from build123d import *

# Parameters (mm, degrees)
SKETCH1_R           = 44.45
BOSS_EXTRUDE1_DEPTH = 10
BOSS_EXTRUDE2_DEPTH = 3
SKETCH3_R           = 5
CUT_EXTRUDE1_DEPTH  = 10
SKETCH4_R           = 5
SKETCH4_R_2         = 3.25
BOSS_EXTRUDE4_DEPTH = 3
CHAMFER1_SIZE       = 0.5


with BuildPart() as part:
    # Sketch1 → Boss-Extrude1 (new body)
    with BuildSketch(Plane(origin=(0, 0, 0), x_dir=(1, 0, 0), z_dir=(0, 1, 0))):
        with Locations(Location((0, 0, 0), (0, 0, 270))):
            Circle(SKETCH1_R)
        with BuildLine():
            ThreePointArc((37.087043144, 17.293972236), (28.935533906, 28.935533906), (17.293972236, 37.087043144))
            ThreePointArc((17.293972236, 37.087043144), (10.649341992, 34.668595517), (13.067789619, 28.023965273))
            ThreePointArc((13.067789619, 28.023965273), (21.864466094, 21.864466094), (28.023965273, 13.067789619))
            ThreePointArc((28.023965273, 13.067789619), (34.668595517, 10.649341992), (37.087043144, 17.293972236))
        make_face(mode=Mode.SUBTRACT)
        with BuildLine():
            ThreePointArc((17.293972236, -37.087043144), (28.935533906, -28.935533906), (37.087043144, -17.293972236))
            ThreePointArc((37.087043144, -17.293972236), (34.668595517, -10.649341992), (28.023965273, -13.067789619))
            ThreePointArc((28.023965273, -13.067789619), (21.864466094, -21.864466094), (13.067789619, -28.023965273))
            ThreePointArc((13.067789619, -28.023965273), (10.649341992, -34.668595517), (17.293972236, -37.087043144))
        make_face(mode=Mode.SUBTRACT)
        with BuildLine():
            ThreePointArc((-37.087043144, -17.293972236), (-28.935533906, -28.935533906), (-17.293972236, -37.087043144))
            ThreePointArc((-17.293972236, -37.087043144), (-10.649341992, -34.668595517), (-13.067789619, -28.023965273))
            ThreePointArc((-13.067789619, -28.023965273), (-21.864466094, -21.864466094), (-28.023965273, -13.067789619))
            ThreePointArc((-28.023965273, -13.067789619), (-34.668595517, -10.649341992), (-37.087043144, -17.293972236))
        make_face(mode=Mode.SUBTRACT)
        with BuildLine():
            ThreePointArc((-17.293972236, 37.087043144), (-28.935533906, 28.935533906), (-37.087043144, 17.293972236))
            ThreePointArc((-37.087043144, 17.293972236), (-34.668595517, 10.649341992), (-28.023965273, 13.067789619))
            ThreePointArc((-28.023965273, 13.067789619), (-21.864466094, 21.864466094), (-13.067789619, 28.023965273))
            ThreePointArc((-13.067789619, 28.023965273), (-10.649341992, 34.668595517), (-17.293972236, 37.087043144))
        make_face(mode=Mode.SUBTRACT)
    extrude(amount=BOSS_EXTRUDE1_DEPTH)

    # Sketch2 → Boss-Extrude2 (add)
    with BuildSketch(Plane(origin=(0, 10, 0), x_dir=(1, 0, 0), z_dir=(0, 1, 0))):
        with BuildLine():
            ThreePointArc((-17.293972236, 37.087043144), (-28.935533906, 28.935533906), (-37.087043144, 17.293972236))
            ThreePointArc((-37.087043144, 17.293972236), (-34.668595517, 10.649341992), (-28.023965273, 13.067789619))
            ThreePointArc((-28.023965273, 13.067789619), (-21.864466094, 21.864466094), (-13.067789619, 28.023965273))
            ThreePointArc((-13.067789619, 28.023965273), (-10.649341992, 34.668595517), (-17.293972236, 37.087043144))
        make_face()
        with BuildLine():
            ThreePointArc((-16.554390278, 35.501004516), (-12.23538062, 33.929013559), (-13.807371577, 29.610003901))
            ThreePointArc((-13.807371577, 29.610003901), (-23.101902961, 23.101902961), (-29.610003901, 13.807371577))
            ThreePointArc((-29.610003901, 13.807371577), (-33.929013559, 12.23538062), (-35.501004516, 16.554390278))
            ThreePointArc((-35.501004516, 16.554390278), (-27.698097039, 27.698097039), (-16.554390278, 35.501004516))
        make_face(mode=Mode.SUBTRACT)
        with BuildLine():
            ThreePointArc((17.293972236, 37.087043144), (10.649341992, 34.668595517), (13.067789619, 28.023965273))
            ThreePointArc((13.067789619, 28.023965273), (21.864466094, 21.864466094), (28.023965273, 13.067789619))
            ThreePointArc((28.023965273, 13.067789619), (34.668595517, 10.649341992), (37.087043144, 17.293972236))
            ThreePointArc((37.087043144, 17.293972236), (28.935533906, 28.935533906), (17.293972236, 37.087043144))
        make_face()
        with BuildLine():
            ThreePointArc((35.501004516, 16.554390278), (33.929013559, 12.23538062), (29.610003901, 13.807371577))
            ThreePointArc((29.610003901, 13.807371577), (23.101902961, 23.101902961), (13.807371577, 29.610003901))
            ThreePointArc((13.807371577, 29.610003901), (12.23538062, 33.929013559), (16.554390278, 35.501004516))
            ThreePointArc((16.554390278, 35.501004516), (27.698097039, 27.698097039), (35.501004516, 16.554390278))
        make_face(mode=Mode.SUBTRACT)
        with BuildLine():
            ThreePointArc((37.087043144, -17.293972236), (34.668595517, -10.649341992), (28.023965273, -13.067789619))
            ThreePointArc((28.023965273, -13.067789619), (21.864466094, -21.864466094), (13.067789619, -28.023965273))
            ThreePointArc((13.067789619, -28.023965273), (10.649341992, -34.668595517), (17.293972236, -37.087043144))
            ThreePointArc((17.293972236, -37.087043144), (28.935533906, -28.935533906), (37.087043144, -17.293972236))
        make_face()
        with BuildLine():
            ThreePointArc((16.554390278, -35.501004516), (12.23538062, -33.929013559), (13.807371577, -29.610003901))
            ThreePointArc((13.807371577, -29.610003901), (23.101902961, -23.101902961), (29.610003901, -13.807371577))
            ThreePointArc((29.610003901, -13.807371577), (33.929013559, -12.23538062), (35.501004516, -16.554390278))
            ThreePointArc((35.501004516, -16.554390278), (27.698097039, -27.698097039), (16.554390278, -35.501004516))
        make_face(mode=Mode.SUBTRACT)
        with BuildLine():
            ThreePointArc((-28.023965273, -13.067789619), (-34.668595517, -10.649341992), (-37.087043144, -17.293972236))
            ThreePointArc((-37.087043144, -17.293972236), (-28.935533906, -28.935533906), (-17.293972236, -37.087043144))
            ThreePointArc((-17.293972236, -37.087043144), (-10.649341992, -34.668595517), (-13.067789619, -28.023965273))
            ThreePointArc((-13.067789619, -28.023965273), (-21.864466094, -21.864466094), (-28.023965273, -13.067789619))
        make_face()
        with BuildLine():
            ThreePointArc((-35.501004516, -16.554390278), (-33.929013559, -12.23538062), (-29.610003901, -13.807371577))
            ThreePointArc((-29.610003901, -13.807371577), (-23.101902961, -23.101902961), (-13.807371577, -29.610003901))
            ThreePointArc((-13.807371577, -29.610003901), (-12.23538062, -33.929013559), (-16.554390278, -35.501004516))
            ThreePointArc((-16.554390278, -35.501004516), (-27.698097039, -27.698097039), (-35.501004516, -16.554390278))
        make_face(mode=Mode.SUBTRACT)
    extrude(amount=-BOSS_EXTRUDE2_DEPTH)

    # Sketch3 → Cut-Extrude1 (cut)
    with BuildSketch(Plane(origin=(0, 10, 0), x_dir=(1, 0, 0), z_dir=(0, 1, 0))):
        with Locations(Location((0, 14.664696837, 0), (0, 0, 270))):
            Circle(SKETCH3_R)
        with Locations(Location((-12.7, -7.332348419, 0), (0, 0, 270))):
            Circle(SKETCH3_R)
        with Locations(Location((12.7, -7.332348419, 0), (0, 0, 270))):
            Circle(SKETCH3_R)
    extrude(amount=-CUT_EXTRUDE1_DEPTH, mode=Mode.SUBTRACT)

    # Sketch4 → Boss-Extrude4 (add)
    with BuildSketch(Plane(origin=(0, 0, 0), x_dir=(1, 0, 0), z_dir=(0, 1, 0))):
        with Locations(Location((12.7, -7.332348419, 0), (0, 0, 270))):
            Circle(SKETCH4_R)
        with Locations(Location((12.7, -7.332348419, 0), (0, 0, 270))):
            Circle(SKETCH4_R_2, mode=Mode.SUBTRACT)
        with Locations(Location((-12.7, -7.332348419, 0), (0, 0, 270))):
            Circle(SKETCH4_R)
        with Locations(Location((-12.7, -7.332348419, 0), (0, 0, 270))):
            Circle(SKETCH4_R_2, mode=Mode.SUBTRACT)
        with Locations(Location((0, 14.664696837, 0), (0, 0, 270))):
            Circle(SKETCH4_R)
        with Locations(Location((0, 14.664696837, 0), (0, 0, 270))):
            Circle(SKETCH4_R_2, mode=Mode.SUBTRACT)
    extrude(amount=BOSS_EXTRUDE4_DEPTH)

    # Chamfer1
    chamfer1_edges = [part.edges().sort_by_distance(p)[0] for p in [
        (-34.668595517, 0, 10.649341992),
        (-28.935533906, 0, 28.935533906),
        (-10.649341992, 0, 34.668595517),
        (-21.864466094, 0, 21.864466094),
        (0, 0, -44.45),
        (10.649341992, 0, 34.668595517),
        (28.935533906, 0, 28.935533906),
        (34.668595517, 0, 10.649341992),
        (21.864466094, 0, 21.864466094),
        (-28.935533906, 0, -28.935533906),
        (-34.668595517, 0, -10.649341992),
        (-21.864466094, 0, -21.864466094),
        (-10.649341992, 0, -34.668595517),
        (34.668595517, 0, -10.649341992),
        (28.935533906, 0, -28.935533906),
        (10.649341992, 0, -34.668595517),
        (21.864466094, 0, -21.864466094),
        (0, 10, -44.45),
    ]]
    chamfer(chamfer1_edges, length=CHAMFER1_SIZE)


solid = part.part
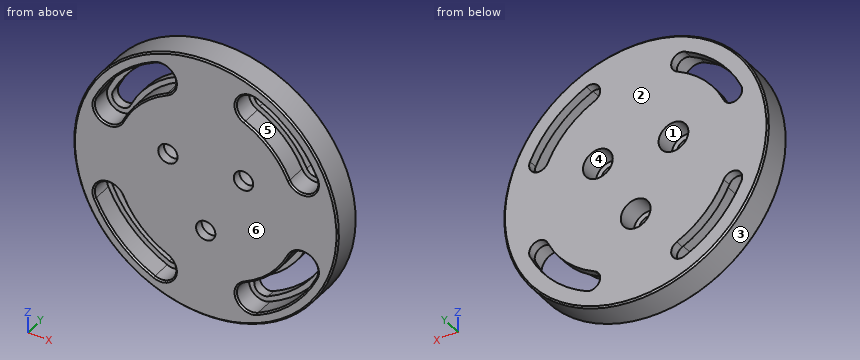
Here's how the part is built. I have some questions about the finished solid (model axes, mm). Face numbers are marked on the shaded views. A direction names the side the tool comes from. Round coordinates to 2 decimals unless told otherwise and drop trailing zeros. Loops run counter-clockwise (first coordinate to the right, second up) from the corner with the lowest first, then second, coordinate; pieces in that order, holes last. Notation, with made-up numbers: (-6, 4.25) - (41, 4.25) arc R23 ccw to (41, 18.25) - close; hole circle Ø6 at (-39.5, 15). An arc over 180 degrees is marked (long way). One line per question, with ' | ' between items. Start each with the question number.
Q1. For the marked faces 4, 5 and 6, which set-ups out of +Z, -Z, +X, -X, +Y, -Y let a thin tool reach every point of the face, with its end or its side?
Q2. I want a section at B-B (x = 0). Write out the boundary of the cut face in (y, z).
Q3. Please list where these lines run through material, in increasing order: line 1 (X direction, y = 4.75, z = 5.5); line 2 (Z direction, x = 14, y = 6.25); line 3 (X direction, y = 2.75, z = 37). Write a range as [from, to].
Q4. I want a section at A-A (y = 4.5). Write out the boundary of the cut face in (x, z), then the cut area to 3 significant figures.
Q5. Will these pins go through, and if not, where does the flat tip stop? pin 1 (3 mm diameter, centred on x = 14.5, z = 5.5, fed in from +Y); pin 2 (3 mm diameter, centred on y = 6, z = 2.5, fed in from +X); pin 3 (3 mm diameter, centred on x = -10.5, y = 2.5, fed in from -Z).
Q6. I want a section at C-C (x = 20). State how many separate pieces and enclosed holes the cut face has, then the cut area to 3 significant figures.
Q7. We'd pull the mould along Z, two halves only. Please class the marked faces 1, 2 and 3: +Z half, -Z half, draft (parallel to the pull), parting line (faces both ways), or undercut.
Response values:
1) face 4: +Y | face 5: -Y | face 6: +Z, -Z, +X, -X, -Y
2) outline: (0, -43.95) - (0.5, -44.45) - (9.5, -44.45) - (10, -43.95) - (10, -19.66) - (3, -19.66) - (3, -17.91) - (0, -17.91) - close; (0, -11.41) - (3, -11.41) - (3, -9.66) - (10, -9.66) - (10, 43.95) - (9.5, 44.45) - (0.5, 44.45) - (0, 43.95) - close
3) line 1: x = [-44.11, -17.35], [-8.05, 8.05], [17.35, 44.11] | line 2: z = [-42.19, -37.41], [-27.57, 2.5], [12.16, 27.57], [37.41, 42.19] | line 3: x = [-24.63, -17.48], [-12.89, 12.89], [17.48, 24.63]
4) outline: circle Ø88.9 at (0, 0); hole (-37.09, -17.29) arc R40.92 ccw to (-17.29, -37.09) arc R5 ccw to (-13.07, -28.02) arc R30.92 cw to (-28.02, -13.07) arc R5 ccw to start; hole (-37.09, 17.29) arc R5 ccw to (-28.02, 13.07) arc R30.92 cw to (-13.07, 28.02) arc R5 ccw to (-17.29, 37.09) arc R40.92 ccw to start; hole circle Ø10 at (-12.7, 7.33); hole circle Ø10 at (0, -14.66); hole circle Ø10 at (12.7, 7.33); hole (13.07, -28.02) arc R5 ccw to (17.29, -37.09) arc R40.92 ccw to (37.09, -17.29) arc R5 ccw to (28.02, -13.07) arc R30.92 cw to start; hole (13.07, 28.02) arc R30.92 cw to (28.02, 13.07) arc R5 ccw to (37.09, 17.29) arc R40.92 ccw to (17.29, 37.09) arc R5 ccw to start | area: 4,650 mm²
5) pin 1: stops at y = 3 | pin 2: stops at x = 44.44 | pin 3: stops at z = -43.53
6) separate pieces: 3 | enclosed holes: 0 | area: 576 mm²
7) face 1: undercut | face 2: draft | face 3: parting line
